Geometry: final body of the model. Coordinates: model frame, mm. A direction names the side the tool comes from. Give positions to 0.01 mm unless a question says otherwise; leave off trailing zeros. Write each loop counter-clockwise with the first axis right and the second up, starting at its lowest first coordinate (ties: lowest second). Pieces come first, ordered by that corner, then holes. Notation, with made-up numbers: (66.5, 34.25) - (94.5, 34.25) arc R3 ccw to (94.5, 38.25) - close; hole circle Ø6 at (73.5, 84). An arc over 180 degrees is marked (long way). Use CSV: the item, a comma, the result in double quotes. Start each with the question number.
(1) Section A-A on x = -5.5. Output: boundary loops of the cut face in (y, z).
(2) Section D-D on x = 0. Output: boundary loops of the cut face in (y, z), and give its area (3 significant figures).
(3) Section C-C on y = 9.75. Output: boundary loops of the cut face in (x, z).
(4) First-contact query: pin 1 Ø12 at (x, y) = (-3, 13) entering from -Z; pin 2 Ø6.5 at (x, z) = (0, 30) entering from -Y; pin 3 Ø0.8 at (x, z) = (7.5, -29) entering from +Y; pin 4 Ø1 at (y, z) = (19.5, -25) entering from -X. Flat tips, straight axial feed; report the tip coordinate or a pass-through.
(5) Section B-B on z = 30. Output: boundary loops of the cut face in (x, y), and give its area (3 significant figures).
(6) Line query: probe 1 along Y at (x, z) = (-0.25, 17.5); probe 2 along X at (y, z) = (16.25, -2); probe 3 along Y at (x, z) = (1.75, 32.5). Output: solid intervals per line, ascending. Write a range as [from, to].
(7) Reachability of faces 4 (the flat face through (0, 18, 0)), 5 (the flat face through (8, 19, -30)), 6 (the cylindrical face through (-1.278, 1.014, -31.666)), 7 (the flat face through (8, 19, 30)) from +Z, -Z, +X, -X, +Y, -Y: full face, straight path, thin tool, end or side. Return the list, or none.
(8) Draft query along Y for faces 1 (the flat face through (0, 20, -1)), 2 (the flat face through (10, 11, 1)), 3 (the flat face through (-7, 10, 0)). Return one class per face: released by +Y, released by -Y, zero draft, split by the parting line, or undercut.
from build123d import *

# Parameters (mm, degrees)
CROQUIS1_W              = 20
CROQUIS1_H              = 80
SALIENTE_EXTRUIR1_DEPTH = 2
CROQUIS2_W              = 3
CROQUIS2_H              = 80
SALIENTE_EXTRUIR2_DEPTH = 16
REDONDEO1_R             = 2
REDONDEO2_R             = 2
CROQUIS3_W              = 20
CROQUIS3_H              = 80
SALIENTE_EXTRUIR3_DEPTH = 2
CROQUIS5_R              = 2.1
CORTAR_EXTRUIR1_DEPTH   = 2
CROQUIS6_W              = 18
CROQUIS6_H              = 20
CORTAR_EXTRUIR3_DEPTH   = 2
CROQUIS7_W              = 3
CROQUIS7_H              = 40
SALIENTE_EXTRUIR4_DEPTH = 16


with BuildPart() as part:
    # Croquis1 → Saliente-Extruir1 (new body)
    with BuildSketch(Plane(origin=(0, 0, 0), x_dir=(1, 0, 0), z_dir=(0, 1, 0))):
        Rectangle(CROQUIS1_W, CROQUIS1_H)
    extrude(amount=SALIENTE_EXTRUIR1_DEPTH)

    # Croquis2 → Saliente-Extruir2 (add)
    with BuildSketch(Plane(origin=(0, 2, 0), x_dir=(1, 0, 0), z_dir=(0, 1, 0))):
        with Locations((8.5, 0)):
            Rectangle(CROQUIS2_W, CROQUIS2_H)
    extrude(amount=SALIENTE_EXTRUIR2_DEPTH)

    # Redondeo1
    redondeo1_edges = [part.edges().sort_by_distance(p)[0] for p in [
        (10, 0, 0),
    ]]
    fillet(redondeo1_edges, radius=REDONDEO1_R)

    # Redondeo2
    redondeo2_edges = [part.edges().sort_by_distance(p)[0] for p in [
        (7, 2, 0),
    ]]
    fillet(redondeo2_edges, radius=REDONDEO2_R)

    # Croquis3 → Saliente-Extruir3 (add)
    with BuildSketch(Plane(origin=(0, 18, 0), x_dir=(1, 0, 0), z_dir=(0, 1, 0))):
        Rectangle(CROQUIS3_W, CROQUIS3_H)
    extrude(amount=SALIENTE_EXTRUIR3_DEPTH)

    # Croquis5 → Cortar-Extruir1 (cut)
    with BuildSketch(Plane(origin=(0, 2, 0), x_dir=(1, 0, 0), z_dir=(0, 1, 0))):
        with Locations(Location((0, 30, 0), (0, 0, 270))):
            Circle(CROQUIS5_R)
        with Locations(Location((0, -30, 0), (0, 0, 270))):
            Circle(CROQUIS5_R)
    extrude(amount=-CORTAR_EXTRUIR1_DEPTH, mode=Mode.SUBTRACT)

    # Croquis6 → Cortar-Extruir3 (cut)
    with BuildSketch(Plane(origin=(0, 20, 0), x_dir=(1, 0, 0), z_dir=(0, 1, 0))):
        with Locations((-1, 30)):
            Rectangle(CROQUIS6_W, CROQUIS6_H)
        with Locations((-1, -30)):
            Rectangle(CROQUIS6_W, CROQUIS6_H)
    extrude(amount=-CORTAR_EXTRUIR3_DEPTH, mode=Mode.SUBTRACT)

    # Croquis7 → Saliente-Extruir4 (add)
    with BuildSketch(Plane(origin=(0, 2, 0), x_dir=(1, 0, 0), z_dir=(0, 1, 0))):
        with Locations((-8.5, 0)):
            Rectangle(CROQUIS7_W, CROQUIS7_H)
    extrude(amount=SALIENTE_EXTRUIR4_DEPTH)


solid = part.part
Check values:
1,outline,"(0, -40) - (2, -40) - (2, 40) - (0, 40) - close; (18, -20) - (20, -20) - (20, 20) - (18, 20) - close"
2,outline,"(0, -40) - (2, -40) - (2, -32.1) - (0, -32.1) - close; (0, -27.9) - (2, -27.9) - (2, 27.9) - (0, 27.9) - close; (0, 32.1) - (2, 32.1) - (2, 40) - (0, 40) - close; (18, -20) - (20, -20) - (20, 20) - (18, 20) - close"
2,area,"223 mm²"
3,outline,"(-10, -20) - (-7, -20) - (-7, 20) - (-10, 20) - close; (7, -40) - (10, -40) - (10, 40) - (7, 40) - close"
4,pin 1,"stops at z = -20"
4,pin 2,"stops at y = 0"
4,pin 3,"stops at y = 18"
4,pin 4,"stops at x = 8"
5,outline,"(-10, 0) - (-2.1, 0) - (-2.1, 2) - (-10, 2) - close; (2.1, 0) - (8, 0) arc R2 ccw to (10, 2) - (10, 20) - (8, 20) - (8, 18) - (7, 18) - (7, 4) arc R2 cw to (5, 2) - (2.1, 2) - close"
5,area,"83.6 mm²"
6,probe 1,"y = [0, 2], [18, 20]"
6,probe 2,"x = [-10, -7], [7, 10]"
6,probe 3,"y = [0, 2]"
7,face 4,"+Z, -Z"
7,face 5,"-Z, -X, +Y"
7,face 6,"+Y, -Y"
7,face 7,"+Z, -X, +Y"
8,face 1,"released by +Y"
8,face 2,"zero draft"
8,face 3,"undercut"
